```python
from build123d import *

# Parameters (mm, degrees)
BOSS_EXTRUDE1_DEPTH     = 8
CUT_EXTRUDE1_DEPTH      = 1
CUT_EXTRUDE1_DEPTH_BACK = 37
CUT_EXTRUDE2_DEPTH      = 1
CUT_EXTRUDE2_DEPTH_BACK = 37
CUT_EXTRUDE6_DEPTH      = 5


with BuildPart() as part:
    # Sketch1 → Boss-Extrude1 (new body)
    with BuildSketch(Plane(origin=(0, 0, 0), x_dir=(1, 0, 0), z_dir=(0, 1, 0))):
        with BuildLine():
            Line((-3, 0), (0, 0))
            Line((0, 0), (0, 22))
            ThreePointArc((0, 22), (-2.121320344, 22.878679656), (-3, 25))
            Line((-3, 25), (-3, 0))
        make_face()
        with BuildLine():
            ThreePointArc((-3, 25), (-2.121320344, 22.878679656), (0, 22))
            Line((0, 22), (0, 22.878679656))
            Line((0, 22.878679656), (0, 25))
            Line((0, 25), (-2.121320344, 27.121320344))
            ThreePointArc((-2.121320344, 27.121320344), (-2.771638598, 26.148050297), (-3, 25))
        make_face()
        with BuildLine():
            ThreePointArc((0, 28), (-1.148050297, 27.771638598), (-2.121320344, 27.121320344))
            Line((-2.121320344, 27.121320344), (0, 25))
            Line((0, 25), (2.121320344, 25))
            Line((2.121320344, 25), (3, 25))
            ThreePointArc((3, 25), (2.121320344, 27.121320344), (0, 28))
        make_face()
        with BuildLine():
            Line((30, 28), (0, 28))
            ThreePointArc((0, 28), (2.121320344, 27.121320344), (3, 25))
            Line((3, 25), (27, 25))
            ThreePointArc((27, 25), (27.878679656, 27.121320344), (30, 28))
        make_face()
        with BuildLine():
            Line((2.121320344, 25), (0, 25))
            Line((0, 25), (0.621320344, 24.378679656))
            ThreePointArc((0.621320344, 24.378679656), (1.309526193, 24.838524104), (2.121320344, 25))
        make_face()
        with BuildLine():
            Line((0, 25), (0, 22.878679656))
            ThreePointArc((0, 22.878679656), (0.161475896, 23.690473807), (0.621320344, 24.378679656))
            Line((0.621320344, 24.378679656), (0, 25))
        make_face()
        with BuildLine():
            Line((27.878679656, 25), (30, 25))
            Line((30, 25), (32.121320344, 27.121320344))
            ThreePointArc((32.121320344, 27.121320344), (31.148050297, 27.771638598), (30, 28))
            ThreePointArc((30, 28), (27.878679656, 27.121320344), (27, 25))
            Line((27, 25), (27.878679656, 25))
        make_face()
        with BuildLine():
            Line((29.378679656, 24.378679656), (30, 25))
            Line((30, 25), (27.878679656, 25))
            ThreePointArc((27.878679656, 25), (28.690473807, 24.838524104), (29.378679656, 24.378679656))
        make_face()
        with BuildLine():
            ThreePointArc((29.378679656, 24.378679656), (29.838524104, 23.690473807), (30, 22.878679656))
            Line((30, 22.878679656), (30, 25))
            Line((30, 25), (29.378679656, 24.378679656))
        make_face()
        with BuildLine():
            Line((30, 22.878679656), (30, 22))
            ThreePointArc((30, 22), (32.121320344, 22.878679656), (33, 25))
            ThreePointArc((33, 25), (32.771638598, 26.148050297), (32.121320344, 27.121320344))
            Line((32.121320344, 27.121320344), (30, 25))
            Line((30, 25), (30, 22.878679656))
        make_face()
        with BuildLine():
            Line((30, 22), (30, 0))
            Line((30, 0), (33, 0))
            Line((33, 0), (33, 25))
            ThreePointArc((33, 25), (32.121320344, 22.878679656), (30, 22))
        make_face()
    extrude(amount=BOSS_EXTRUDE1_DEPTH)

    # Sketch2 → Cut-Extrude1 (cut, two sides)
    with BuildSketch(Plane.ZY.offset(3)) as cut_extrude1_sk:
        with BuildLine():
            ThreePointArc((-5.13137085, 5.13137085), (-5.13137085, 2.86862915), (-2.86862915, 2.86862915))
            Line((-2.86862915, 2.86862915), (-5.13137085, 5.13137085))
        make_face()
        with BuildLine():
            Line((-5.13137085, 5.13137085), (-2.86862915, 2.86862915))
            ThreePointArc((-2.86862915, 2.86862915), (-2.521792748, 3.387706508), (-2.4, 4))
            ThreePointArc((-2.4, 4), (-3.387706508, 5.478207252), (-5.13137085, 5.13137085))
        make_face()
    extrude(amount=CUT_EXTRUDE1_DEPTH, mode=Mode.SUBTRACT)
    extrude(cut_extrude1_sk.sketch, amount=-CUT_EXTRUDE1_DEPTH_BACK, mode=Mode.SUBTRACT)

    # Sketch3 → Cut-Extrude2 (cut, two sides)
    with BuildSketch(Plane.ZY.offset(3)) as cut_extrude2_sk:
        with BuildLine():
            Line((0, 0), (-2.868629152, 0))
            Line((-2.86862915, 0), (-2.86862915, -3.234663016))
            ThreePointArc((-2.86862915, -3.234663016), (2.247050128, -1.115679278), (4.366033866, 4))
            ThreePointArc((4.366033866, 4), (2.247050128, 9.115679278), (-2.86862915, 11.234663016))
            Line((-2.86862915, 11.234663016), (-2.86862915, 8))
            Line((-2.86862915, 8), (0, 8))
            Line((0, 8), (0, 5.13137085))
            Line((0, 5.13137085), (0, 2.86862915))
            Line((0, 2.86862915), (0, 0))
        make_face()
        with BuildLine():
            ThreePointArc((0, 2.86862915), (-0.840202026, 0.840202025), (-2.868629152, 0))
            Line((-2.868629152, 0), (0, 0))
            Line((0, 0), (0, 2.86862915))
        make_face()
        with BuildLine():
            Line((0, 8), (-2.86862915, 8))
            ThreePointArc((-2.86862915, 8), (-0.840202025, 7.159797975), (0, 5.13137085))
            Line((0, 5.13137085), (0, 8))
        make_face()
    extrude(amount=CUT_EXTRUDE2_DEPTH, mode=Mode.SUBTRACT)
    extrude(cut_extrude2_sk.sketch, amount=-CUT_EXTRUDE2_DEPTH_BACK, mode=Mode.SUBTRACT)

    # Sketch4 → Cut-Extrude6 (cut)
    with BuildSketch(Plane(origin=(0, 0, -28), x_dir=(-1, 0, 0), z_dir=(0, 0, -1))):
        with BuildLine():
            ThreePointArc((-13.5, 4), (-13.512715795, 4.194899187), (-13.550647591, 4.386493976))
            Line((-13.550647591, 4.386493976), (-16.449352409, 3.613506024))
            ThreePointArc((-16.449352409, 3.613506024), (-14.805100813, 2.512715795), (-13.5, 4))
        make_face()
        with BuildLine():
            Line((-16.449352409, 3.613506024), (-13.550647591, 4.386493976))
            ThreePointArc((-13.550647591, 4.386493976), (-15.386493976, 5.449352409), (-16.449352409, 3.613506024))
        make_face()
    extrude(amount=-CUT_EXTRUDE6_DEPTH, mode=Mode.SUBTRACT)


solid = part.part
```
Can you work these out from the model? Positions are in its coordinate system, mm. A direction names the side the tool comes from. Round coordinates to 2 decimals unless told otherwise and drop trailing zeros. Loops run counter-clockwise (first coordinate to the right, second up) from the corner with the lowest first, then second, coordinate; pieces in that order, holes last.
Item 1: Will this pin go through, and if not, where does the flat tip stop? pin 1 Ø1 at (x, y) = (14.5, 5) entering from +Z.
Item 2: Suppose I cut it at C-C, the plane x = 3. Write out the boundary of the cut face in (y, z).
Item 3: Suppose I cut it at B-B, the plane z = -4. Write out the boundary of the cut face in (x, y).
Item 4: Which directions (+Z, -Z, +X, -X, +Y, -Y) give clear straight access to the entire face, cutting with the end or side of a thin tool? Please do faces 5 (the flat face through (15, 2, -28)), 6 (the flat face through (15, 2, -25)).
Item 5: If we mould it in two halves opening along X, with no side actions, what happens to faces 1 (the flat face through (-3, 4, -13)), 2 (the flat face through (31, 4, 0)), 3 (the flat face through (33, 4, -12)), 4 (the flat face through (0, 4, -11))? For each: +X half, -X half, draft (parallel to the pull), parting line (faces both ways), or undercut.
Item 6: Please list where these lines run through material, in increasing order: L1, parallel to X at y = 6.75, z = -17.25; L2, parallel to Z at x = 13, y = 2; L3, parallel to X at y = 5, z = -25.5.
Item 7: Suppose I cut it at D-D, the plane y = 2. Write out the boundary of the cut face in (x, z), then the cut area to 3 significant figures.
Item 8: Suppose I cut it at A-A, the plane z = -19.75. Write out the boundary of the cut face in (x, y), then the cut area to 3 significant figures.
Reported:
1. pin 1: stops at z = -25
2. outline: (0, -28) - (8, -28) - (8, -25) - (0, -25) - close
3. outline: (-3, 0) - (0, 0) - (0, 2.4) - (-3, 2.4) - close; (-3, 5.6) - (0, 5.6) - (0, 8) - (-3, 8) - close; (30, 0) - (33, 0) - (33, 2.4) - (30, 2.4) - close; (30, 5.6) - (33, 5.6) - (33, 8) - (30, 8) - close
4. face 5: -Z, +X, -X, +Y, -Y
4. face 6: +Z, +Y, -Y
5. face 1: -X half
5. face 2: draft
5. face 3: +X half
5. face 4: undercut
6. L1: x = -3 to 0, 30 to 33
6. L2: z = -28 to -25
6. L3: x = -2.96 to 13.88, 16.12 to 32.96
7. outline: (-3, -25) arc R3 ccw to (0, -28) - (30, -28) arc R3 ccw to (33, -25) - (33, -0.13) - (30, -0.13) - (30, -22.88) arc R2.12 cw to (27.88, -25) - (2.12, -25) arc R2.12 cw to (0, -22.88) - (0, -0.13) - (-3, -0.13) - close
7. area: 255 mm2
8. outline: (-3, 0) - (0, 0) - (0, 8) - (-3, 8) - close; (30, 0) - (33, 0) - (33, 8) - (30, 8) - close
8. area: 48.0 mm2
